Model file for the job. Use its own axes, mm. A direction names the side the tool comes from. Coordinates: 2 decimals unless noted, no trailing zeros. Write item = value, one per line. Start each with the question number.
from build123d import *

# Parameters (mm, degrees)
PAD_DEPTH       = 15
SKETCH001_R     = 10
PAD001_DEPTH    = 2
FILLET_R        = 2
POCKET_DEPTH    = 1.25
POCKET001_DEPTH = 1
FILLET001_R     = 1
CHAMFER_SIZE    = 0.75


with BuildPart() as part:
    # Sketch → Pad (new body)
    with BuildSketch(Plane.XY):
        Polygon((7.5, 0), (6.761481, 1.811733), (6.495191, 3.75), (4.949747, 4.949747), (3.75, 6.495191), (1.811733, 6.761481), (0, 7.5), (-1.811733, 6.761481), (-3.75, 6.495191), (-4.949747, 4.949747), (-6.495191, 3.75), (-6.761481, 1.811733), (-7.5, 0), (-6.761481, -1.811733), (-6.495191, -3.75), (-4.949747, -4.949747), (-3.75, -6.495191), (-1.811733, -6.761481), (0, -7.5), (1.811733, -6.761481), (3.75, -6.495191), (4.949747, -4.949747), (6.495191, -3.75), (6.761481, -1.811733), align=None)
    extrude(amount=PAD_DEPTH)

    # Sketch001 (on Face25 of Pad) → Pad001 (join)
    with BuildSketch(Plane(origin=(0, 0, 0), x_dir=(1, 0, 0), z_dir=(0, 0, -1))):
        Circle(SKETCH001_R)
    extrude(amount=PAD001_DEPTH)

    # Fillet
    fillet_edges = [part.edges().sort_by_distance(p)[0] for p in [
        (7.13074, 0.905867, 15),
        (6.628336, 2.780867, 15),
        (5.722469, 4.349874, 15),
        (4.349874, 5.722469, 15),
        (2.780867, 6.628336, 15),
        (0.905867, 7.13074, 15),
        (-0.905867, 7.13074, 15),
        (-2.780867, 6.628336, 15),
        (-4.349874, 5.722469, 15),
        (-5.722469, 4.349874, 15),
        (-6.628336, 2.780867, 15),
        (-7.13074, 0.905867, 15),
        (-7.13074, -0.905867, 15),
        (-6.628336, -2.780867, 15),
        (-5.722469, -4.349874, 15),
        (-4.349874, -5.722469, 15),
        (-2.780867, -6.628336, 15),
        (-0.905867, -7.13074, 15),
        (0.905867, -7.13074, 15),
        (2.780867, -6.628336, 15),
        (4.349874, -5.722469, 15),
        (5.722469, -4.349874, 15),
        (6.628336, -2.780867, 15),
        (7.13074, -0.905867, 15),
        (-3.75, -6.495191, 7.5),
        (-1.811733, -6.761481, 7.5),
        (0, -7.5, 7.5),
        (1.811733, -6.761481, 7.5),
        (3.75, -6.495191, 7.5),
        (4.949747, -4.949747, 7.5),
        (6.495191, -3.75, 7.5),
        (6.761481, -1.811733, 7.5),
        (7.5, 0, 7.5),
        (6.761481, 1.811733, 7.5),
        (6.495191, 3.75, 7.5),
        (4.949747, 4.949747, 7.5),
        (3.75, 6.495191, 7.5),
        (1.811733, 6.761481, 7.5),
        (0, 7.5, 7.5),
        (-1.811733, 6.761481, 7.5),
        (-3.75, 6.495191, 7.5),
        (-4.949747, 4.949747, 7.5),
        (-6.495191, 3.75, 7.5),
        (-6.761481, 1.811733, 7.5),
        (-7.5, 0, 7.5),
        (-6.761481, -1.811733, 7.5),
        (-6.495191, -3.75, 7.5),
        (-4.949747, -4.949747, 7.5),
    ]]
    fillet(fillet_edges, radius=FILLET_R)

    # Sketch002 (on Face54 of Fillet) → Pocket (cut)
    with BuildSketch(Plane.XY.offset(15)):
        with BuildLine():
            Line((7.192259, 0.754949), (0, 0.754949))
            Line((0, 0.754949), (0, -0.754949))
            Line((0, -0.754949), (7.192259, -0.754949))
            ThreePointArc((7.192259, -0.754949), (7.340219, 0), (7.192259, 0.754949))
        make_face()
    extrude(amount=-POCKET_DEPTH, mode=Mode.SUBTRACT)

    # Sketch003 (on DatumPlane) → Pocket001 (cut)
    with BuildSketch(Plane(origin=(7.790651, 0, 6.5), x_dir=(0, 1, 0), z_dir=(1, 0, 0))):
        Polygon((-0.75, 6.5), (-0.75, -6.5), (0.75, -6.5), (0.75, 6.5), (0.75, 7.25), (-0.75, 7.25), align=None)
    extrude(amount=-POCKET001_DEPTH, mode=Mode.SUBTRACT)

    # Fillet001
    fillet001_edges = [part.edges().sort_by_distance(p)[0] for p in [
        (6.790651, 0, 13.75),
    ]]
    fillet(fillet001_edges, radius=FILLET001_R)

    # Chamfer
    chamfer_edges = [part.edges().sort_by_distance(p)[0] for p in [
        (-10, 0, 0),
    ]]
    chamfer(chamfer_edges, length=CHAMFER_SIZE)


solid = part.part
(1) 3-axis set-ups, long thin cutter, end or side, ignore diameter. For faces 1 (the face through (-1.161, 7.027, 6.409)), 2 (the face through (-7.34, -0.01, 6.59)), 3 (the face through (-7.027, -1.161, 6.409)), 4 (the face through (7, 0, 0)), 5 (the face through (3, 0, 13.75)): which of +Z, -Z, +X, -X, +Y, -Y reach the whole face in a straight line?
(2) Drill centre lines: line 1 along Z through (x, y) = (-8.25, -1.25); line 2 along Y through (x, z) = (4.25, 7); line 3 along Y through (x, z) = (0, 3.5). Where is each one in solid material? Low to high.
(3) Mould opens along Y. For faces 6 (the face through (0, 0, 14)), 7 (the face through (6.362, -3.661, 6.591)), 8 (the face through (-5.155, 4.068, 14.399)) say: released by +Y, released by -Y, zero draft, split by the parting line, or undercut.
(4) Drop flat-ended pins along their axis: pin 1 Ø5 at (x, z) = (-2.5, 7) entering from +Y; pin 2 Ø3 at (x, z) = (7, 7) entering from -Y; pin 3 Ø5 at (x, z) = (-4.5, 6.5) entering from -Y. Give the stop position or say it passes through.
Returned:
q1.face_1 = +Z, -X, +Y
q1.face_2 = +Z, -X
q1.face_3 = +Z, -X, -Y
q1.face_4 = +Z
q1.face_5 = +Z, +X
q2.line_1 = -2 to 0
q2.line_2 = -5.85 to 5.85
q2.line_3 = -7.34 to 7.34
q3.face_6 = undercut
q3.face_7 = released by -Y
q3.face_8 = released by +Y
q4.pin_1 = 7.34
q4.pin_2 = -4.52
q4.pin_3 = -6.74
